Input: part model. Units: mm. Frame: model coordinates. A direction names the side the tool comes from. Give positions to 0.01 mm unless a question says otherwise; leave off trailing zeros. Order: outer loops, then holes, each group sorted by start corner. A loop starts at its lowest first (then second) coordinate and runs counter-clockwise, first axis right, second up. Notation, with made-up numbers: (9.25, 33) - (22.25, 33) arc R29 cw to (22.25, 55) - close; hole circle Ø5 at (-28, -24.5). An arc over 180 degrees is marked (long way). Answer in a Markdown table with one row per item. Add a question column.
from build123d import *

# Parameters (mm, degrees)
F0_W     = 50.8
F0_H     = 50.8
F1_DEPTH = 7.62
F2_T     = -1.27
F4_DEPTH = 25.4


with BuildPart() as f1:
    # F0 (on Top) → F1 (new body)
    with BuildSketch(Plane.XY):
        with Locations((-25.4, 25.4)):
            Rectangle(F0_W, F0_H)
    extrude(amount=F1_DEPTH)

    # F2
    f2_openings = [f1.faces().sort_by_distance(p)[0] for p in [
        (-25.4, 25.4, 7.62),
    ]]
    offset(amount=F2_T, openings=f2_openings)

    # F3 (on face) → F4 (cut)
    with BuildSketch(Plane.XY.offset(1.27)):
        with BuildLine():
            ThreePointArc((-45.569412, 11.43), (-47.737438, 12.328026), (-46.839412, 10.16))
            ThreePointArc((-46.839412, 10.16), (-45.941387, 10.531974), (-45.569412, 11.43))
        make_face()
        with BuildLine():
            ThreePointArc((-46.839412, 5.08), (-48.109412, 3.81), (-46.839412, 2.54))
            Line((-46.839412, 2.54), (-46.839412, 3.81))
            Line((-46.839412, 3.81), (-46.839412, 5.08))
        make_face()
        with BuildLine():
            Line((-46.839412, 3.81), (-46.839412, 2.54))
            ThreePointArc((-46.839412, 2.54), (-45.941387, 2.911974), (-45.569412, 3.81))
            ThreePointArc((-45.569412, 3.81), (-45.941387, 4.708026), (-46.839412, 5.08))
            Line((-46.839412, 5.08), (-46.839412, 3.81))
        make_face()
    extrude(amount=-F4_DEPTH, mode=Mode.SUBTRACT)


solid = f1.part
Q1. Section A-A, the plane z = 2.25. Return loops of the section in (x, y), then the cut area to 3 significant figures.
Q2. Access query for faces 1 (the flat face through (-1.27, 25, 4)), 2 (the flat face through (-26, 26, 0)). Directions: +Z, -Z, +X, -X, +Y, -Y. A direction counts if a zero-diameter tool reaches every point of the face in a straight line with its end or side. Return the directions, or none.
Q3. Section C-C, the plane y = 45. Return loops of the section in (x, z), then the cut area to 3 significant figures.
Q4. Line query: probe 1 along X at (y, z) = (11.43, 0.8); probe 2 along Y at (x, z) = (-29, 7.5); probe 3 along X at (y, z) = (13.5, 4). Output: solid intervals per line, ascending.
Q5. Pull-direction query (X, two-part tool) for faces 3 (the flat face through (-26, 1.27, 4)), 4 (the flat face through (0, 25, 4)), 5 (the flat face through (-50.8, 25, 4)), 6 (the flat face through (-27, 1, 7.62)); classes: +X half, -X half, draft (parallel to the pull), parting line (faces both ways), or undercut.
Q6. Section B-B, the plane x = -38.5. Return loops of the section in (y, z), then the cut area to 3 significant figures.
Computed:
| question | item | result |
|---|---|---|
| 1 | outline | (-50.8, 0) - (0, 0) - (0, 50.8) - (-50.8, 50.8) - close; hole (-49.53, 1.27) - (-1.27, 1.27) - (-1.27, 49.53) - (-49.53, 49.53) - close |
| 1 | area | 252 mm^2 |
| 2 | face 1 | +Z |
| 2 | face 2 | -Z, +X, -X, +Y, -Y |
| 3 | outline | (-50.8, 0) - (0, 0) - (0, 7.62) - (-1.27, 7.62) - (-1.27, 1.27) - (-49.53, 1.27) - (-49.53, 7.62) - (-50.8, 7.62) - close |
| 3 | area | 80.6 mm^2 |
| 4 | probe 1 | x = -50.8 to -48.11, -45.57 to 0 |
| 4 | probe 2 | y = 0 to 1.27, 49.53 to 50.8 |
| 4 | probe 3 | x = -50.8 to -49.53, -1.27 to 0 |
| 5 | face 3 | undercut |
| 5 | face 4 | +X half |
| 5 | face 5 | -X half |
| 5 | face 6 | draft |
| 6 | outline | (0, 0) - (50.8, 0) - (50.8, 7.62) - (49.53, 7.62) - (49.53, 1.27) - (1.27, 1.27) - (1.27, 7.62) - (0, 7.62) - close |
| 6 | area | 80.6 mm^2 |
